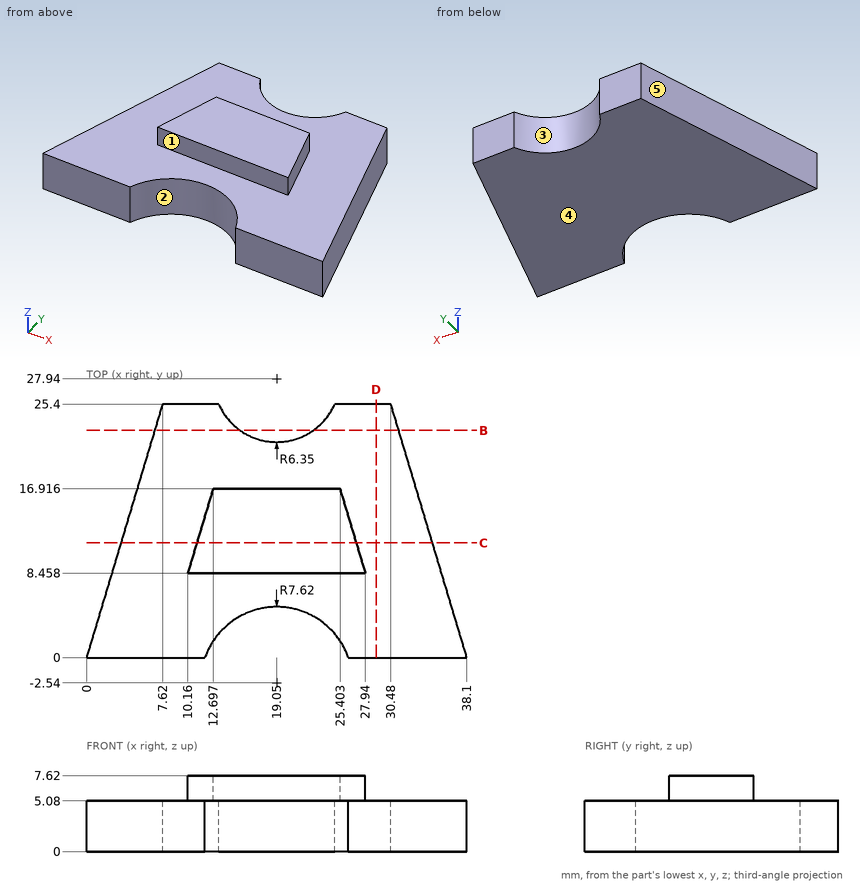
Part print with two shaded views. Sizes in mm from the minimum x, y, z corner. A direction names the side the tool comes from. Coordinates: 2 decimals unless noted, no trailing zeros. Order: outer loops, then holes, each group sorted by start corner. A loop starts at its lowest first (then second) coordinate and runs counter-clockwise, first axis right, second up. Notation, with made-up numbers: (0.25, 80.5) - (57.25, 80.5) arc R21 cw to (57.25, 90.5) - close; hole circle Ø1 at (55, 48). An arc over 180 degrees is marked (long way). Write item = value, one per line. Start each with the question number.
1) Saw through at C-C on y = 11.5. Write the cut outline in (x, z).
2) Wall check: line 1 along Z through (x, y) = (2.5, 5.5); line 2 along X through (y, z) = (4, 1.75); line 3 along Y through (x, z) = (18, 6.75). Give the ranges that are in metal, low to high. Write a range as from..to.
3) Saw through at B-B on y = 22.75. Write the cut outline in (x, z) (1 decimal).
4) Saw through at D-D on x = 29. Write the cut outline in (y, z), then the cut area to 3 significant figures.
5) Two-plate mould, pull along X, no slides. Class the marked faces 3, 4 and 5: pulls with the +X half, pulls with the -X half, needs draft (parallel to the pull), parting line crosses it, or undercut.
6) Flat gauge pins, fed straight in: pin 1 Ø2 at (x, z) = (22, 6.5) entering from +Y; pin 2 Ø4 at (y, z) = (12.5, 3.5) entering from -X; pin 3 Ø2 at (y, z) = (3.5, 1.5) entering from -X. Where does each tip first touch, or does it go through?
7) 3-axis set-ups, long thin cutter, end or side, ignore diameter. For the marked faces 1 and 2: which of +Z, -Z, +X, -X, +Y, -Y reach the whole face in a straight line?
From the geometry:
q1.outline = (3.45, 0) - (34.65, 0) - (34.65, 5.08) - (27.03, 5.08) - (27.03, 7.62) - (11.07, 7.62) - (11.07, 5.08) - (3.45, 5.08) - close
q2.line_1 = 0..5.08
q2.line_2 = 1.2..15.14, 22.96..36.9
q2.line_3 = 8.46..16.92
q3.outline = (6.8, 0) - (15.4, 0) - (15.4, 5.1) - (6.8, 5.1) - close; (22.7, 0) - (31.3, 0) - (31.3, 5.1) - (22.7, 5.1) - close
q4.outline = (0, 0) - (25.4, 0) - (25.4, 5.08) - (0, 5.08) - close
q4.area = 129 mm^2
q5.face_3 = undercut
q5.face_4 = needs draft
q5.face_5 = pulls with the -X half
q6.pin_1 = 16.92
q6.pin_2 = 3.15
q6.pin_3 = 0.75
q7.face_1 = +Z, +X, -X, -Y
q7.face_2 = +Z, -Z, -Y
